```python
from build123d import *

# Parameters (mm, degrees)
SKETCH1_W                = 31
SKETCH1_H                = 22
BOSS_EXTRUDE1_DEPTH      = 11
SKETCH3_W                = 24.5
SKETCH3_H                = 15.5
CUT_EXTRUDE1_DEPTH       = 7.75
FILLET1_R                = 7.75
CUT_EXTRUDE2_DEPTH       = 32.812929761
CUT_EXTRUDE2_DEPTH_BACK  = 32.812929761
SKETCH4_R                = 5
SKETCH5_W                = 8
SKETCH5_H                = 8
SKETCH5_R                = 1.905800151
BOSS_EXTRUDE3_DEPTH      = 6
MIRROR9_COPY_1_SKETCH_W  = 8
MIRROR9_COPY_1_SKETCH_H  = 8
MIRROR9_COPY_1_SKETCH_R  = 1.905800151
MIRROR9_COPY_1_DEPTH     = 6
CUT_EXTRUDE4_START       = -2
SKETCH7_R                = 1.905800151
CUT_EXTRUDE4_DEPTH       = 2
MIRROR11_START           = -2
MIRROR11_COPY_1_SKETCH_R = 1.905800151
MIRROR11_COPY_1_DEPTH    = 2
CHAMFER3_SIZE            = 4


with BuildPart() as part:
    # Sketch1 → Boss-Extrude1 (new body)
    with BuildSketch(Plane(origin=(0, 0, 0), x_dir=(1, 0, 0), z_dir=(0, 1, 0))):
        Rectangle(SKETCH1_W, SKETCH1_H)
    extrude(amount=BOSS_EXTRUDE1_DEPTH)

    # Sketch3 → Cut-Extrude1 (cut)
    with BuildSketch(Plane(origin=(0, 11, 0), x_dir=(1, 0, 0), z_dir=(0, 1, 0))):
        Rectangle(SKETCH3_W, SKETCH3_H)
    extrude(amount=-CUT_EXTRUDE1_DEPTH, mode=Mode.SUBTRACT)

    # Fillet1
    fillet1_edges = [part.edges().sort_by_distance(p)[0] for p in [
        (0, 3.25, 7.75),
        (0, 3.25, -7.75),
    ]]
    fillet(fillet1_edges, radius=FILLET1_R - 0.0001)  # a hair under: the kernel refuses the full size

    # Sketch4 → Cut-Extrude2 (cut, two sides: drawn at the far end of the back side and taken through both)
    with BuildSketch(Plane(origin=(-12.25, 0, 0), x_dir=(0, 0, -1), z_dir=(1, 0, 0)).offset(-CUT_EXTRUDE2_DEPTH_BACK)):
        with Locations((0, 11)):
            Circle(SKETCH4_R)
    extrude(amount=CUT_EXTRUDE2_DEPTH + CUT_EXTRUDE2_DEPTH_BACK, mode=Mode.SUBTRACT)

    # Sketch5 → Boss-Extrude3 (add)
    with BuildSketch(Plane(origin=(0, 11, 0), x_dir=(1, 0, 0), z_dir=(0, 1, 0))):
        with Locations((11.5, -15)):
            Rectangle(SKETCH5_W, SKETCH5_H)
        with Locations(Location((11.5, -15, 0), (0, 0, 270))):
            Circle(SKETCH5_R, mode=Mode.SUBTRACT)
    boss_extrude3 = extrude(amount=-BOSS_EXTRUDE3_DEPTH)

    # Mirror8: Boss-Extrude3 across plane
    add(boss_extrude3.mirror(Plane(origin=(0, 0, 0), x_dir=(0, 0, 1), z_dir=(1, 0, 0))))

    # Mirror9: Boss-Extrude3 across plane
    add(boss_extrude3.mirror(Plane.XY))

    # Mirror9 copy 1 sketch → Mirror9 copy 1 (add)
    with BuildSketch(Plane(origin=(0, 11, 0), x_dir=(-1, 0, 0), z_dir=(0, 1, 0))):
        with Locations((11.5, -15)):
            Rectangle(MIRROR9_COPY_1_SKETCH_W, MIRROR9_COPY_1_SKETCH_H)
        with Locations(Location((11.5, -15, 0), (0, 0, 270))):
            Circle(MIRROR9_COPY_1_SKETCH_R, mode=Mode.SUBTRACT)
    extrude(amount=-MIRROR9_COPY_1_DEPTH)

    # Sketch7 → Cut-Extrude4 (cut)
    with BuildSketch(Plane.XZ.offset(-5).offset(CUT_EXTRUDE4_START)):
        Polygon((14.675426481, 15), (13.08771324, 17.75), (9.91228676, 17.75), (8.324573519, 15), (9.91228676, 12.25), (13.08771324, 12.25), align=None)
        with Locations(Location((11.5, 15, 0), (0, 0, 90))):
            Circle(SKETCH7_R, mode=Mode.SUBTRACT)
    cut_extrude4 = extrude(amount=CUT_EXTRUDE4_DEPTH, mode=Mode.SUBTRACT)

    # Mirror10: Cut-Extrude4 across plane
    add(cut_extrude4.mirror(Plane(origin=(0, 0, 0), x_dir=(0, 0, 1), z_dir=(1, 0, 0))), mode=Mode.SUBTRACT)

    # Mirror11: Cut-Extrude4 across plane
    add(cut_extrude4.mirror(Plane.XY), mode=Mode.SUBTRACT)

    # Mirror11 copy 1 sketch → Mirror11 copy 1 (cut)
    with BuildSketch(Plane(origin=(0, 5, 0), x_dir=(-1, 0, 0), z_dir=(0, -1, 0)).offset(MIRROR11_START)):
        Polygon((14.675426481, 15), (13.08771324, 17.75), (9.91228676, 17.75), (8.324573519, 15), (9.91228676, 12.25), (13.08771324, 12.25), align=None)
        with Locations(Location((11.5, 15, 0), (0, 0, 90))):
            Circle(MIRROR11_COPY_1_SKETCH_R, mode=Mode.SUBTRACT)
    extrude(amount=MIRROR11_COPY_1_DEPTH, mode=Mode.SUBTRACT)

    # Chamfer3
    chamfer3_edges = [part.edges().sort_by_distance(p)[0] for p in [
        (7.5, 8, 11),
        (-7.5, 8, 11),
        (-7.5, 8, -11),
        (7.5, 8, -11),
    ]]
    chamfer(chamfer3_edges, length=CHAMFER3_SIZE)


solid = part.part
```
CAD build for the part. Positions are in the model's coordinates, mm. A direction names the side the tool comes from. Coordinates: 2 decimals unless noted, no trailing zeros. Order: outer loops, then holes, each group sorted by start corner. A loop starts at its lowest first (then second) coordinate and runs counter-clockwise, first axis right, second up. Notation, with made-up numbers: (31, 80) -> (70, 80) arc R11 cw to (70, 98) -> close; hole circle Ø6 at (-8, 29). An arc over 180 degrees is marked (long way). Use one line per item in the form item = value. Start each with the question number.
1) Drop flat-ended pins along their axis: pin 1 (4 mm diameter, centred on y = 8.5, z = -1, fed in from -X); pin 2 (1.6 mm diameter, centred on x = -13, z = 15, fed in from -Y); pin 3 (1 mm diameter, centred on x = -4, y = 2, fed in from -Z); pin 4 (4 mm diameter, centred on x = -1.5, y = 4, fed in from +Z). Give the stop position or say it passes through.
2) Band-saw the part on A-A on y = 9.25. State how many separate pieces and enclosed holes the cut face has, then the cut area to 3 significant figures.
3) Drill centre lines: L1, parallel to X at y = 6.75, z = -3; L2, parallel to Z at x = 11.5, y = 9.85; L3, parallel to Z at x = -11.5, y = 9.1. Where is each one in solid material? Low to high. Write a range as [from, to].
4) Band-saw the part on D-D on z = -1.5. Give the cut face in (x, y), then the cut area to 3 significant figures.
5) Pull direction X, two halves, no side cores. Call faces 4 (the flat face through (0, 11, 10)), 5 (the flat face through (13.87, 6.014, 13.606)), 6 (the flat face through (15.5, 5.6, -0.3)): +X half, -X half, draft (parallel to the pull), parting line (faces both ways), or undercut.
6) Tool access for faces 1 (the flat face through (-11, 6, 12.25)), 2 (the flat face through (5.5, 8, 13)), 3 (the flat face through (12.25, 5, 0)): list every direction of +Z, -Z, +X, -X, +Y, -Y with a clear straight run to the whole face (end or side of a thin tool).
Entries:
q1.pin_1 = through
q1.pin_2 = 7
q1.pin_3 = -11
q1.pin_4 = 11
q2.separate_pieces = 2
q2.enclosed_holes = 4
q2.area = 494 mm2
q3.L1 = [-15.5, -12.25], [12.25, 15.5]
q3.L2 = [-19, -16.91], [-13.09, -7.66], [7.66, 13.09], [16.91, 19]
q3.L3 = [-19, -16.91], [-13.09, -7.51], [7.51, 13.09], [16.91, 19]
q4.outline = (-15.5, 0) -> (15.5, 0) -> (15.5, 6.23) -> (12.25, 6.23) -> (12.25, 3.4) -> (-12.25, 3.4) -> (-12.25, 6.23) -> (-15.5, 6.23) -> close
q4.area = 124 mm2
q5.face_4 = draft
q5.face_5 = undercut
q5.face_6 = +X half
q6.face_1 = -Y
q6.face_2 = +Z, +Y, -Y
q6.face_3 = +Y
